Input: part model. Units: mm. Frame: model coordinates. A direction names the side the tool comes from. Round coordinates to 2 decimals unless told otherwise and drop trailing zeros. Loops run counter-clockwise (first coordinate to the right, second up) from the corner with the lowest first, then second, coordinate; pieces in that order, holes last. Notation, with made-up numbers: (60.5, -26) -> (71.5, -26) arc R22 cw to (71.5, 0) -> close; hole circle Ø9 at (-34.75, -18.75). An arc over 180 degrees is marked (long way). Answer as a JSON object with one key per item and string values.
```python
from build123d import *

# Parameters (mm, degrees)
SKETCH1_W                           = 40
SKETCH1_H                           = 10
BOSS_EXTRUDE1_DEPTH                 = 10
M4X0_7_TAPPED_HOLE1_D               = 3.3
M4X0_7_TAPPED_HOLE1_DEPTH           = 16
M4X0_7_TAPPED_HOLE1_TIP             = 0.991420021
M4X0_7_TAPPED_HOLE1_ON_FACE_2_D     = 3.3
M4X0_7_TAPPED_HOLE1_ON_FACE_2_DEPTH = 16
M4X0_7_TAPPED_HOLE1_ON_FACE_2_TIP   = 0.991420021


with BuildPart() as part:
    # Sketch1 → Boss-Extrude1 (new body)
    with BuildSketch(Plane(origin=(0, 0, 0), x_dir=(1, 0, 0), z_dir=(0, 1, 0))):
        Rectangle(SKETCH1_W, SKETCH1_H)
    extrude(amount=BOSS_EXTRUDE1_DEPTH)

    # M4x0.7 Tapped Hole1
    with Locations(Plane(origin=(-20, 5, 0), x_dir=(0, 0, -1), z_dir=(-1, 0, 0))):
        with Locations((0, 0)):
            Hole(M4X0_7_TAPPED_HOLE1_D / 2, depth=M4X0_7_TAPPED_HOLE1_DEPTH)
            with Locations((0, 0, -(M4X0_7_TAPPED_HOLE1_DEPTH + M4X0_7_TAPPED_HOLE1_TIP / 2))):  # 118° drill point
                Cone(0, M4X0_7_TAPPED_HOLE1_D / 2, M4X0_7_TAPPED_HOLE1_TIP, mode=Mode.SUBTRACT)

    # M4x0.7 Tapped Hole1 on face 2
    with Locations(Plane(origin=(20, 5, 0), x_dir=(0, 0, 1), z_dir=(1, 0, 0))):
        with Locations((0, 0)):
            Hole(M4X0_7_TAPPED_HOLE1_ON_FACE_2_D / 2, depth=M4X0_7_TAPPED_HOLE1_ON_FACE_2_DEPTH)
            with Locations((0, 0, -(M4X0_7_TAPPED_HOLE1_ON_FACE_2_DEPTH + M4X0_7_TAPPED_HOLE1_ON_FACE_2_TIP / 2))):  # 118° drill point
                Cone(0, M4X0_7_TAPPED_HOLE1_ON_FACE_2_D / 2, M4X0_7_TAPPED_HOLE1_ON_FACE_2_TIP, mode=Mode.SUBTRACT)


solid = part.part
```
1) Reachability of faces 1 (the face through (0, 0, 0)), 2 (the face through (11.9, 6.6, 0.4)), 3 (the face through (-11.9, 6.6, -0.4)) from +Z, -Z, +X, -X, +Y, -Y: full face, straight path, thin tool, end or side. Return the list, or none.
Output:
{"face 1": "+Z, -Z, +X, -X, -Y", "face 2": "+X", "face 3": "-X"}
2) Contact query for a flat-ended pin moving along its axis: P1, Ø2, axis at y = 5, z = 0, coming from the -X side. Output: stop coordinate, or through.
Output:
{"P1": "stops at x = -3.61"}
3) Draft query along Y for faces 4 (the face through (3.2, 5.3, 0.1)), 5 (the face through (20, 3, 0)), 6 (the face through (-3.2, 5.3, -0.1)), 7 (the face through (0, 10, 0)). Return one class per face: +Y half, -Y half, draft (parallel to the pull), parting line (faces both ways), or undercut.
Output:
{"face 4": "undercut", "face 5": "draft", "face 6": "undercut", "face 7": "+Y half"}
4) Ray query, probe 1 along Z at (x, y) = (9.5, 5); probe 2 along Y at (x, z) = (7, 0); probe 3 along Y at (x, z) = (-15.5, 1.25). Return the intervals inside material, ascending.
Output:
{"probe 1": "z = -5 to -1.65, 1.65 to 5", "probe 2": "y = 0 to 3.35, 6.65 to 10", "probe 3": "y = 0 to 3.92, 6.08 to 10"}
5) Section A-A, the plane x = 10. Output: boundary loops of the cut face in (y, z).
Output:
{"outline": "(0, -5) -> (10, -5) -> (10, 5) -> (0, 5) -> close; hole circle Ø3.3 at (5, 0)"}
